Verification items for the finished model (mm, model axes). A direction names the side the tool comes from. Give positions to 0.01 mm unless a question says otherwise; leave off trailing zeros. Write each loop counter-clockwise with the first axis right and the second up, starting at its lowest first coordinate (ties: lowest second). Pieces come first, ordered by that corner, then holes. Notation, with made-up numbers: (-33, 14) -> (15, 14) arc R29 ccw to (15, 39) -> close; hole circle Ø4 at (47, -0.75). An arc over 180 degrees is marked (long way). Write item = value, one per line.
from build123d import *

# Parameters (mm, degrees)
SKETCH1_W           = 431.8
SKETCH1_H           = 95.25
BOSS_EXTRUDE1_DEPTH = 6.35
SKETCH2_W           = 12.7
SKETCH2_H           = 6.35
CUT_EXTRUDE1_DEPTH  = 443.226327801
LPATTERN1_COUNT     = 17
LPATTERN1_PITCH     = 25.4
SKETCH3_W           = 6.35
SKETCH3_H           = 6.35
CUT_EXTRUDE2_DEPTH  = 443.226327801
SKETCH5_W           = 6.35
SKETCH5_H           = 12.7
CUT_EXTRUDE4_DEPTH  = 443.226327801
LPATTERN2_COUNT     = 2
LPATTERN2_PITCH     = 25.4
LPATTERN2_COL_COUNT = 2
LPATTERN2_COL_PITCH = 25.4
SKETCH6_W           = 114.3
SKETCH6_H           = 46.0375
CUT_EXTRUDE5_DEPTH  = 443.226327801
SKETCH7_R           = 1.75
CUT_EXTRUDE6_DEPTH  = 443.226327801
SKETCH8_W           = 6.35
SKETCH8_H           = 9.525
SKETCH8_H_2         = 12.7
CUT_EXTRUDE7_DEPTH  = 443.226327801
LPATTERN3_COUNT     = 2
LPATTERN3_PITCH     = 425.45
SKETCH9_W           = 304.8
SKETCH9_H           = 95.25
CUT_EXTRUDE8_DEPTH  = 443.226327801
SKETCH10_W          = 6.35
SKETCH10_H          = 15.875
CUT_EXTRUDE9_DEPTH  = 443.226327801
SKETCH11_W          = 57.65
SKETCH11_H          = 19.05
CUT_EXTRUDE10_DEPTH = 443.226327801
SKETCH12_W          = 63.5
SKETCH12_H          = 25.4
CUT_EXTRUDE11_DEPTH = 443.226327801
SKETCH13_W          = 19.05
SKETCH13_H          = 19.05
CUT_EXTRUDE12_DEPTH = 443.226327801
SKETCH14_W          = 33.6
SKETCH14_H          = 6.35
CUT_EXTRUDE13_DEPTH = 443.226327801
FILLET1_R           = 6.35
FILLET2_R           = 6.35
FILLET3_R           = 2.54


with BuildPart() as part:
    # Sketch1 → Boss-Extrude1 (new body)
    with BuildSketch(Plane(origin=(0, 0, 0), x_dir=(1, 0, 0), z_dir=(0, 1, 0))):
        with Locations((215.9, 47.625)):
            Rectangle(SKETCH1_W, SKETCH1_H)
    extrude(amount=BOSS_EXTRUDE1_DEPTH)

    # Sketch2 → Cut-Extrude1 (cut, through all)
    with BuildSketch(Plane(origin=(0, 6.35, 0), x_dir=(1, 0, 0), z_dir=(0, 1, 0))):
        with Locations((12.7, 92.075)):
            Rectangle(SKETCH2_W, SKETCH2_H)
        with Locations((12.7, 3.175)):
            Rectangle(SKETCH2_W, SKETCH2_H)
    cut_extrude1 = extrude(amount=-CUT_EXTRUDE1_DEPTH, mode=Mode.SUBTRACT)

    # LPattern1: Cut-Extrude1 ×17
    with Locations(*[(i * LPATTERN1_PITCH, 0, 0) for i in range(1, LPATTERN1_COUNT)]):
        add(cut_extrude1, mode=Mode.SUBTRACT)

    # Sketch3 → Cut-Extrude2 (cut, through all)
    with BuildSketch(Plane(origin=(0, 6.35, 0), x_dir=(1, 0, 0), z_dir=(0, 1, 0))):
        with Locations((3.175, 92.075)):
            Rectangle(SKETCH3_W, SKETCH3_H)
        with Locations((3.175, 3.175)):
            Rectangle(SKETCH3_W, SKETCH3_H)
        with Locations((428.625, 92.075)):
            Rectangle(SKETCH3_W, SKETCH3_H)
        with Locations((428.625, 3.175)):
            Rectangle(SKETCH3_W, SKETCH3_H)
    extrude(amount=-CUT_EXTRUDE2_DEPTH, mode=Mode.SUBTRACT)

    # Sketch5 → Cut-Extrude4 (cut, through all)
    with BuildSketch(Plane(origin=(0, 6.35, 0), x_dir=(1, 0, 0), z_dir=(0, 1, 0))):
        with Locations((187.325, 47.625)):
            Rectangle(SKETCH5_W, SKETCH5_H)
        with Locations((307.975, 47.625)):
            Rectangle(SKETCH5_W, SKETCH5_H)
    cut_extrude4 = extrude(amount=-CUT_EXTRUDE4_DEPTH, mode=Mode.SUBTRACT)

    # LPattern2: Cut-Extrude4 ×2
    with Locations(*[(0, 0, -i * LPATTERN2_PITCH) for i in range(1, LPATTERN2_COUNT)]):
        add(cut_extrude4, mode=Mode.SUBTRACT)

    # LPattern2 col: Cut-Extrude4 ×2
    with Locations(*[(0, 0, i * LPATTERN2_COL_PITCH) for i in range(1, LPATTERN2_COL_COUNT)]):
        add(cut_extrude4, mode=Mode.SUBTRACT)

    # Sketch6 → Cut-Extrude5 (cut, through all)
    with BuildSketch(Plane(origin=(0, 6.35, 0), x_dir=(1, 0, 0), z_dir=(0, 1, 0))):
        with Locations((247.65, 47.625)):
            Rectangle(SKETCH6_W, SKETCH6_H)
    extrude(amount=-CUT_EXTRUDE5_DEPTH, mode=Mode.SUBTRACT)

    # Sketch7 → Cut-Extrude6 (cut, through all)
    with BuildSketch(Plane(origin=(0, 6.35, 0), x_dir=(1, 0, 0), z_dir=(0, 1, 0))):
        with Locations(Location((52.65, 44.45, 0), (0, 0, 270))):
            Circle(SKETCH7_R)
        with Locations(Location((116.65, 44.45, 0), (0, 0, 270))):
            Circle(SKETCH7_R)
        with Locations(Location((315.15, 44.45, 0), (0, 0, 270))):
            Circle(SKETCH7_R)
        with Locations(Location((379.15, 44.45, 0), (0, 0, 270))):
            Circle(SKETCH7_R)
    extrude(amount=-CUT_EXTRUDE6_DEPTH, mode=Mode.SUBTRACT)

    # Sketch8 → Cut-Extrude7 (cut, through all)
    with BuildSketch(Plane(origin=(0, 6.35, 0), x_dir=(1, 0, 0), z_dir=(0, 1, 0))):
        with Locations((3.175, 84.1375)):
            Rectangle(SKETCH8_W, SKETCH8_H)
        with Locations((3.175, 11.1125)):
            Rectangle(SKETCH8_W, SKETCH8_H)
        with Locations((3.175, 34.925)):
            Rectangle(SKETCH8_W, SKETCH8_H_2)
        with Locations((3.175, 60.325)):
            Rectangle(SKETCH8_W, SKETCH8_H_2)
    cut_extrude7 = extrude(amount=-CUT_EXTRUDE7_DEPTH, mode=Mode.SUBTRACT)

    # LPattern3: Cut-Extrude7 ×2
    with Locations(*[(i * LPATTERN3_PITCH, 0, 0) for i in range(1, LPATTERN3_COUNT)]):
        add(cut_extrude7, mode=Mode.SUBTRACT)

    # Sketch9 → Cut-Extrude8 (cut, through all)
    with BuildSketch(Plane(origin=(0, 6.35, 0), x_dir=(1, 0, 0), z_dir=(0, 1, 0))):
        with Locations((152.4, 47.625)):
            Rectangle(SKETCH9_W, SKETCH9_H)
    extrude(amount=-CUT_EXTRUDE8_DEPTH, mode=Mode.SUBTRACT)

    # Sketch10 → Cut-Extrude9 (cut, through all)
    with BuildSketch(Plane(origin=(0, 6.35, 0), x_dir=(1, 0, 0), z_dir=(0, 1, 0))):
        with Locations((307.975, 87.3125)):
            Rectangle(SKETCH10_W, SKETCH10_H)
        with Locations((307.975, 7.9375)):
            Rectangle(SKETCH10_W, SKETCH10_H)
    extrude(amount=-CUT_EXTRUDE9_DEPTH, mode=Mode.SUBTRACT)

    # Sketch11 → Cut-Extrude10 (cut, through all)
    with BuildSketch(Plane(origin=(0, 6.35, 0), x_dir=(1, 0, 0), z_dir=(0, 1, 0))):
        with Locations((347.15, 73.025)):
            Rectangle(SKETCH11_W, SKETCH11_H)
    extrude(amount=-CUT_EXTRUDE10_DEPTH, mode=Mode.SUBTRACT)

    # Sketch12 → Cut-Extrude11 (cut, through all)
    with BuildSketch(Plane(origin=(0, 6.35, 0), x_dir=(1, 0, 0), z_dir=(0, 1, 0))):
        with Locations((387.35, 25.4)):
            Rectangle(SKETCH12_W, SKETCH12_H)
    extrude(amount=-CUT_EXTRUDE11_DEPTH, mode=Mode.SUBTRACT)

    # Sketch13 → Cut-Extrude12 (cut, through all)
    with BuildSketch(Plane(origin=(0, 6.35, 0), x_dir=(1, 0, 0), z_dir=(0, 1, 0))):
        with Locations((327.025, 22.225)):
            Rectangle(SKETCH13_W, SKETCH13_H)
    extrude(amount=-CUT_EXTRUDE12_DEPTH, mode=Mode.SUBTRACT)

    # Sketch14 → Cut-Extrude13 (cut, through all)
    with BuildSketch(Plane(origin=(0, 6.35, 0), x_dir=(1, 0, 0), z_dir=(0, 1, 0))):
        with Locations((402.3, 41.275)):
            Rectangle(SKETCH14_W, SKETCH14_H)
    extrude(amount=-CUT_EXTRUDE13_DEPTH, mode=Mode.SUBTRACT)

    # Fillet1
    fillet1_edges = [part.edges().sort_by_distance(p)[0] for p in [
        (385.5, 3.175, -38.1),
    ]]
    fillet(fillet1_edges, radius=FILLET1_R - 0.0001)  # a hair under: the kernel refuses the full size

    # Fillet2
    fillet2_edges = [part.edges().sort_by_distance(p)[0] for p in [
        (385.5, 3.175, -44.45),
    ]]
    fillet(fillet2_edges, radius=FILLET2_R)

    # Fillet3
    fillet3_edges = [part.edges().sort_by_distance(p)[0] for p in [
        (318.325, 3.175, -63.5),
        (318.325, 3.175, -82.55),
        (375.975, 3.175, -82.55),
        (375.975, 3.175, -63.5),
        (419.1, 3.175, -12.7),
        (355.6, 3.175, -12.7),
        (355.6, 3.175, -38.1),
        (317.5, 3.175, -12.7),
        (317.5, 3.175, -31.75),
        (336.55, 3.175, -31.75),
        (336.55, 3.175, -12.7),
        (419.1, 3.175, -44.45),
    ]]
    fillet(fillet3_edges, radius=FILLET3_R)


solid = part.part
Item 1: Sectioned sample at C-C on x = 364.5. Record the cut outline in (y, z), then the cut area to 3 significant figures.
Response values:
outline = (0, -88.9) -> (6.35, -88.9) -> (6.35, -82.55) -> (0, -82.55) -> close; (0, -63.5) -> (6.35, -63.5) -> (6.35, -38.1) -> (0, -38.1) -> close; (0, -12.7) -> (6.35, -12.7) -> (6.35, -6.35) -> (0, -6.35) -> close
area = 242 mm^2
Item 2: Set-up check for faces 5 (the flat face through (336.55, 3, -92)), 6 (the flat face through (394, 3, -6.35)), 7 (the flat face through (429, 3, -41.275)), 8 (the flat face through (317.5, 3, -22)): record each of +Z, -Z, +X, -X, +Y, -Y from which the full face is reachable in a straight line by a thin tool's end or side.
Response values:
face_5 = -Z, +Y, -Y
face_6 = +Z, +Y, -Y
face_7 = +X, +Y, -Y
face_8 = +Y, -Y
Item 3: Material ranges on line 1 (X direction, y = 2.75, z = -24.5); line 2 (Z direction, x = 324.5, y = 4); line 3 (Z direction, x = 379.15, y = 1.5), recorded low to high.
Response values:
line_1 = 311.15 to 317.5, 336.55 to 355.6, 419.1 to 431.8
line_2 = -95.25 to -82.55, -63.5 to -31.75, -12.7 to 0
line_3 = -95.25 to -46.2, -42.7 to -38.1, -12.7 to 0
Item 4: Sectioned sample at B-B on x = 315.15. Record the cut outline in (y, z).
Response values:
outline = (0, -88.9) -> (6.35, -88.9) -> (6.35, -46.2) -> (0, -46.2) -> close; (0, -42.7) -> (6.35, -42.7) -> (6.35, -6.35) -> (0, -6.35) -> close
Item 5: Sectioned sample at D-D on y = 1.5. Give the number of separate pieces and of enclosed holes in the cut face, then the cut area to 3 significant figures.
Response values:
separate_pieces = 1
enclosed_holes = 5
area = 7,190 mm^2
Item 6: Go/stop test with flat-tipped pins: P1, Ø3, axis at y = 4, z = -92.5, coming from the -X side; P2, Ø3, axis at y = 2.5, z = -36.5, coming from the +X side; P3, Ø1.5, axis at x = 373.5, y = 4.5, coming from the -Z side. Record where each tip stops, or that it passes through.
Response values:
P1 = 323.85
P2 = 425.45
P3 = -88.9
Item 7: Sectioned sample at A-A on z = -18.5. Record the cut outline in (x, y).
Response values:
outline = (311.15, 0) -> (317.5, 0) -> (317.5, 6.35) -> (311.15, 6.35) -> close; (336.55, 0) -> (355.6, 0) -> (355.6, 6.35) -> (336.55, 6.35) -> close; (419.1, 0) -> (431.8, 0) -> (431.8, 6.35) -> (419.1, 6.35) -> close
Item 8: Mould release check, pull along Z, two halves, no side actions. Record for faces 1 (the flat face through (356, 3, -95.25)), 2 (the flat face through (327, 3, -12.7)), 3 (the flat face through (336.55, 3, -22)), 4 (the flat face through (367, 0, -48)): +Z half, -Z half, draft (parallel to the pull), parting line (faces both ways), or undercut.
Response values:
face_1 = -Z half
face_2 = undercut
face_3 = undercut
face_4 = draft
